Model file for the job. Use its own axes, mm. A direction names the side the tool comes from. Coordinates: 2 decimals unless noted, no trailing zeros. Loops run counter-clockwise (first coordinate to the right, second up) from the corner with the lowest first, then second, coordinate; pieces in that order, holes last.
from build123d import *

# Parameters (mm, degrees)
F3_R     = 1.6
F4_DEPTH = 25
F5_R     = 2.775
F6_DEPTH = 5


with BuildPart() as f2:
    # F0 (on Top) → F2 (revolve)
    with BuildSketch(Plane.XY):
        Polygon((12.5, 3), (12.5, 0), (25, 0), (25, 10), (20, 10), align=None)
    revolve(axis=Axis((0, 29.101241, 0), (0, 1, 0)))

    # F3 (on face) → F4 (cut)
    with BuildSketch(Plane.XZ):
        with Locations((0, 20)):
            Circle(F3_R)
        with Locations((-17.320508, -10)):
            Circle(F3_R)
        with Locations((17.320508, -10)):
            Circle(F3_R)
    extrude(amount=-F4_DEPTH, mode=Mode.SUBTRACT)

    # F5 (on face) → F6 (cut)
    with BuildSketch(Plane(origin=(0, 10, 0), x_dir=(-1, 0, 0), z_dir=(0, 1, 0))):
        with Locations((0, 20)):
            Circle(F5_R)
        with Locations((-17.320508, -10)):
            Circle(F5_R)
        with Locations((17.320508, -10)):
            Circle(F5_R)
    extrude(amount=-F6_DEPTH, mode=Mode.SUBTRACT)


solid = f2.part
Q1. Which spindle directions (+Z, -Z, +X, -X, +Y, -Y) get a long thin tool onto all of the face, cutting with end or side? Do faces 1 (the flat face through (-19, 5, -11)), 2 (the cylindrical face through (18.06, 2.46, -11.42)). Say none if no direction does.
Answers:
face 1: +Y
face 2: +Y, -Y
Q2. Flat gauge pins, fed straight in: P1, Ø6, axis at x = -8.5, y = 5, coming from the -Z side; P2, Ø3, axis at x = 0.5, z = 21, coming from the +Y side; P3, Ø5, axis at x = -10, z = 9, coming from the +Y side; P4, Ø4.5, axis at x = -17.32, z = -10, coming from the -Y side. Where does each tip first touch, or does it go through?
Answers:
P1: stops at z = -24.39
P2: stops at y = 5
P3: stops at y = 6.22
P4: stops at y = 0
Q3. Slice it at C-C (y = 4.25). List the corners of the cut face in (x, z).
Answers:
outline: circle Ø50 at (0, 0); hole circle Ø3.2 at (-17.32, -10); hole circle Ø27.68 at (0, 0); hole circle Ø3.2 at (0, 20); hole circle Ø3.2 at (17.32, -10)
Q4. Slice it at B-B (x = 0). List the corners of the cut face in (y, z) (3 decimals).
Answers:
outline: (0, -25) - (10, -25) - (10, -20) - (3, -12.5) - (0, -12.5) - close; (0, 12.5) - (3, 12.5) - (7.41, 17.225) - (5, 17.225) - (5, 18.4) - (0, 18.4) - close; (0, 21.6) - (5, 21.6) - (5, 22.775) - (10, 22.775) - (10, 25) - (0, 25) - close
Q5. Mould opens along Z. For faces 3 (the flat face through (-19, 10, 7)), 4 (the cylindrical face through (23.846, 5.07, -7.509)), 5 (the cylindrical face through (-17.67, 2.46, -11.56)) say: +Z half, -Z half, draft (parallel to the pull), parting line (faces both ways), or undercut.
Answers:
face 3: draft
face 4: parting line
face 5: undercut
Q6. Drill centre lines: line 1 (Z direction, x = 0, y = 2.2); line 2 (Z direction, x = 2, y = 6.5); line 3 (X direction, y = 1.1, z = 0). Where is each one in solid material? Low to high.
Answers:
line 1: z = -25 to -12.5, 12.5 to 18.4, 21.6 to 25
line 2: z = -24.92 to -16.13, 16.13 to 18.08, 21.92 to 24.92
line 3: x = -25 to -12.5, 12.5 to 25
Q7. Slice it at D-D (z = -9). Count the separate pieces of the cut face and the enclosed holes in it, and give its area (3 significant figures).
Answers:
separate pieces: 4
enclosed holes: 0
area: 157 mm2
Q8. Slice it at A-A (z = 0). List the corners of the cut face in (x, y), and give its area (4 significant figures).
Answers:
outline: (-25, 0) - (-12.5, 0) - (-12.5, 3) - (-20, 10) - (-25, 10) - close; (12.5, 0) - (25, 0) - (25, 10) - (20, 10) - (12.5, 3) - close
area: 197.5 mm2
